For this review, take the finished solid that the model builds, in its own axes (mm). A direction names the side the tool comes from. Coordinates: 2 decimals unless noted, no trailing zeros. Write each loop counter-clockwise with the first axis right and the second up, starting at its lowest first coordinate (ties: lowest second). Pieces come first, ordered by that corner, then holes. Notation, with made-up numbers: (36.25, 88) - (81.25, 88) arc R27 ccw to (81.25, 106) - close; hole circle Ø10 at (78.25, 43.5). An arc over 180 degrees is marked (long way). Write each question's results on one line, items separated by ' | '.
Autodesk Inventor part; units mm, degrees
ref_plane "YZ Plane" through (0, 0, 0) normal (1, 0, 0) x (0, 1, 0)
ref_plane "XZ Plane" through (0, 0, 0) normal (0, 1, 0) x (-1, 0, 0)
ref_plane "XY Plane" through (0, 0, 0) normal (0, 0, 1) x (1, 0, 0)
sketch "スケッチ1" plane through (0, 0, 0) normal (1, 0, 0) x (0, 1, 0)
  line L0 (0, 0) -> (45, 0)
  line L1 (45, 0) -> (45, 10)
  line L2 (45, 10) -> (0, 10)
  line L3 (0, 10) -> (0, 0)
  line L4 (0, 0) -> (15, 0)
  line L5 (15, 0) -> (15, 30)
  line L6 (15, 30) -> (0, 30)
  line L7 (0, 30) -> (0, 0)
  point P0 (0, 10)
  point P1 (15, 10)
  dimension "d0" = 10
  dimension "d1" = 15
  dimension "d2" = 30
  dimension "d3" = 30
extrude "押し出し1" add sketch "スケッチ1" along normal blind 2
sketch "スケッチ2" plane through (2, 0, 0) normal (1, 0, 0) x (0, 0, -1)
  line L0 (-30, 15) -> (-30, 0)
  line L1 (-30, 7.5) -> (0, 7.5) construction
  line L2 (0, 0) -> (0, 45)
  line L3 (0, 45) -> (-10, 45)
  line L4 (-5, 45) -> (-5, 0) construction
  line L5 (-30, 0) -> (0, 0)
  point P0 (-25, 7.5)
  point P1 (-5, 7.5)
  point P2 (-5, 20)
  point P3 (-5, 40)
  dimension "d6" = 20
  dimension "d7" = 5
  dimension "d8" = 20
  dimension "d9" = 5
hole "穴1" at (2, 7.5, 25) at (2, 7.5, 5) at (2, 20, 5) at (2, 40, 5) direction (-1, 0, 0) diameter 3.2 end through all
properties part number "FrameJointL1510" material "アルミニウム 6061"
Q1. Take a section at A-A on z = 5. State the section outline as (x, y) points.
Results found:
outline: (0, 0) - (2, 0) - (2, 5.9) - (0, 5.9) - close; (0, 9.1) - (2, 9.1) - (2, 18.4) - (0, 18.4) - close; (0, 21.6) - (2, 21.6) - (2, 38.4) - (0, 38.4) - close; (0, 41.6) - (2, 41.6) - (2, 45) - (0, 45) - close
Q2. Mouldability with a two-part tool opening along Z and no side actions: class faces 3 (the face through (1, 22, 0)), 4 (the face through (0.986, 18.414, 5.208)), 5 (the face through (1, 45, 5)), 6 (the face through (0.99, 9.06, 5.35)) as pulls with the +Z half, pulls with the -Z half, needs draft (parallel to the pull), parting line crosses it, or undercut.
Results found:
face 3: pulls with the -Z half | face 4: undercut | face 5: needs draft | face 6: undercut
Q3. Wall thickness on line 1 along Z through (x, y) = (1.05, 7.5); line 2 along Y through (x, z) = (1.65, 5); line 3 along Z through (x, y) = (0.5, 40): over which ranges is each line inside the solid? List them lowest first. Write a range as from..to.
Results found:
line 1: 0..3.4, 6.6..23.4, 26.6..30 | line 2: 0..5.9, 9.1..18.4, 21.6..38.4, 41.6..45 | line 3: 0..3.4, 6.6..10
Q4. Take a section at B-B on z = 25. State the section outline as (x, y) points, plus the area to 3 significant figures.
Results found:
outline: (0, 0) - (2, 0) - (2, 5.9) - (0, 5.9) - close; (0, 9.1) - (2, 9.1) - (2, 15) - (0, 15) - close | area: 23.6 mm2
Q5. For faces 1 (the face through (1, 15, 20)), 2 (the face through (0, 17, 9)), list the 3-axis set-ups (+Z, -Z, +X, -X, +Y, -Y) from which the entire face can be reached by the end or side of a thin tool; tool diameter is ignored.
Results found:
face 1: +Z, +X, -X, +Y | face 2: +Z, -Z, -X, +Y, -Y
Q6. Take a section at C-C on y = 20. State the section outline as (x, z) points.
Results found:
outline: (0, 0) - (2, 0) - (2, 3.4) - (0, 3.4) - close; (0, 6.6) - (2, 6.6) - (2, 10) - (0, 10) - close
Q7. For pin 1 (1 mm diameter, centred on x = 1, y = 31, fed in from +Z); pin 2 (1 mm diameter, centred on x = 1, z = 20.5, fed in from +Y), all flat-tipped, find the tip position at first contact; note any pin that passes through.
Results found:
pin 1: z = 10 | pin 2: y = 15
Q8. Take a section at D-D on y = 7.5. State the section outline as (x, z) points, plus the area to 3 significant figures.
Results found:
outline: (0, 0) - (2, 0) - (2, 3.4) - (0, 3.4) - close; (0, 6.6) - (2, 6.6) - (2, 23.4) - (0, 23.4) - close; (0, 26.6) - (2, 26.6) - (2, 30) - (0, 30) - close | area: 47.2 mm2
